Autodesk Inventor part; units mm, degrees
ref_plane "Work Plane1" through (5, 0, 0) normal (1, 0, 0) x (0, 1, 0)
ref_plane "YZ Plane" through (0, 0, 0) normal (1, 0, 0) x (0, 1, 0)
ref_plane "XZ Plane" through (0, 0, 0) normal (0, 1, 0) x (-1, 0, 0)
ref_plane "Work Plane1" through (5, 0, 0) normal (1, 0, 0) x (0, 1, 0)
sketch "Sketch1" plane through (5, 0, 0) normal (1, 0, 0) x (0, 1, 0)
  line L0 (-72.5, 60) -> (72.5, 60)
  line L1 (72.5, 60) -> (72.5, -60)
  line L2 (72.5, -60) -> (-72.5, -60)
  line L3 (-72.5, -60) -> (-72.5, 60)
  line L4 (-72.5, 60) -> (72.5, -60) construction
  line L5 (72.5, 60) -> (-72.5, -60) construction
  point P0 (0, 0)
  dimension "d0" = 145
  dimension "d1" = 120
extrude "Extrusion1" add sketch "Sketch1" along normal blind 49
shell "Shell2" thickness 2 removed faces 1 at (21.3333, -24.1667, 60)
properties part number "Case"
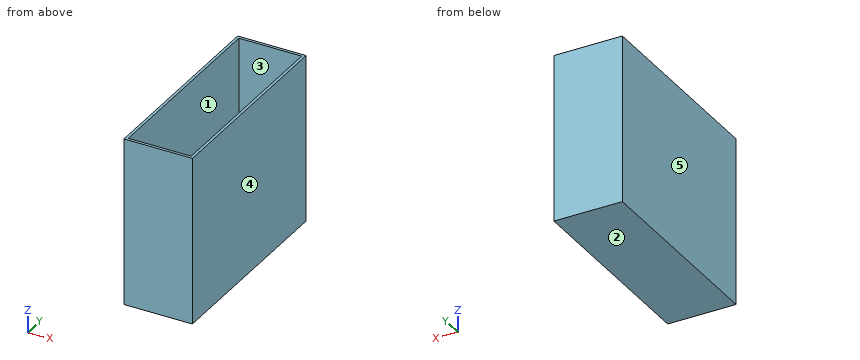
Check sheet for the modelled part. Datum: model origin and axes. Units: mm. Face numbers are marked on the shaded views. A direction names the side the tool comes from. Round coordinates to 2 decimals unless told otherwise and drop trailing zeros. Loops run counter-clockwise (first coordinate to the right, second up) from the corner with the lowest first, then second, coordinate; pieces in that order, holes last. Notation, with made-up numbers: (45.5, 73.5) -> (99.5, 73.5) arc R13 cw to (99.5, 95.5) -> close; hole circle Ø2 at (65, 23.25). An arc over 180 degrees is marked (long way). Put each result on its own line as item: value. Start each with the question number.
1. Section check B-B (x = 33). Enter the section's corners in (y, z).
2. Scan lines: probe 1 along X at (y, z) = (7.5, -52.5); probe 2 along Y at (x, z) = (41, -4.5); probe 3 along Z at (x, y) = (10.5, 30). Record each from-to range of solid material in increasing order.
3. Draft check along X on the marked faces 3, 4 and 5. Enter one of: +X half, -X half, draft (parallel to the pull), parting line (faces both ways), or undercut.
4. Access from +Z, -Z, +X, -X, +Y, -Y to the whole of each face (thin tool, end or side, straight path). Record for the marked faces 1 and 2.
5. Section check C-C (y = 41.5). Enter the section's corners in (x, z).
6. Section check A-A (z = 14.5). Enter the section's corners in (x, y), plus the area to 3 significant figures.
Findings:
1. outline: (-72.5, -60) -> (72.5, -60) -> (72.5, 60) -> (70.5, 60) -> (70.5, -58) -> (-70.5, -58) -> (-70.5, 60) -> (-72.5, 60) -> close
2. probe 1: x = 5 to 7, 52 to 54
2. probe 2: y = -72.5 to -70.5, 70.5 to 72.5
2. probe 3: z = -60 to -58
3. face 3: undercut
3. face 4: +X half
3. face 5: -X half
4. face 1: +Z
4. face 2: -Z, +X, -X, +Y, -Y
5. outline: (5, -60) -> (54, -60) -> (54, 60) -> (52, 60) -> (52, -58) -> (7, -58) -> (7, 60) -> (5, 60) -> close
6. outline: (5, -72.5) -> (54, -72.5) -> (54, 72.5) -> (5, 72.5) -> close; hole (7, -70.5) -> (52, -70.5) -> (52, 70.5) -> (7, 70.5) -> close
6. area: 760 mm^2
